Geometry: final body of the model. Coordinates: model frame, mm. A direction names the side the tool comes from. Coordinates: 2 decimals unless noted, no trailing zeros. Loops run counter-clockwise (first coordinate to the right, second up) from the corner with the lowest first, then second, coordinate; pieces in that order, holes last. Notation, with made-up numbers: (64, 52) -> (89, 52) arc R9 cw to (89, 64) -> close; hole circle Ø9 at (-16, 85). An arc over 180 degrees is marked (long way). One line per item, written item: value. Start each with the question number.
Item 1: Ray query, probe 1 along Y at (x, z) = (-123.5, -20.5) (1 decimal); probe 2 along Z at (x, y) = (-161, 75.5) (3 decimals); probe 3 along Y at (x, z) = (-197, 39) (1 decimal). Return the intervals inside material, ascending. Write a range as from..to.
Item 2: Set-up query: faces 5 (the flat face through (-121, 0, -2)), 6 (the flat face through (-190.5, 285, 1)), 7 (the flat face through (0, 237, -113)). Return all of +Z, -Z, +X, -X, +Y, -Y with unobstructed straight access to the full face (end or side cutting, diameter ignored); none if empty.
Item 3: Contact query for a flat-ended pin moving along its axis: pin 1 Ø3 at (y, z) = (298, 58) entering from +X. Output: stop coordinate, or through.
Item 4: Mould query, pull axis Y, two halves, no side actions, for faces 1 (the cylindrical face through (-143.266, 389.237, 132.457)), 2 (the flat face through (-137, 186, 139.7)), 3 (the flat face through (-122, 201, 104.775)), 4 (the flat face through (-247.65, 110, 1)). Classes: +Y half, -Y half, draft (parallel to the pull), parting line (faces both ways), or undercut.
Item 5: Section query B-B on y = 210. Return loops of the section in (x, z) (3 decimals), then the cut area to 3 significant figures.
Autodesk Inventor part; units mm, degrees
ref_plane "YZ Plane" through (0, 0, 0) normal (1, 0, 0) x (0, 1, 0)
ref_plane "XZ Plane" through (0, 0, 0) normal (0, 1, 0) x (-1, 0, 0)
ref_plane "XY Plane" through (0, 0, 0) normal (0, 0, 1) x (1, 0, 0)
sketch "Sketch1" plane through (0, 0, 0) normal (1, 0, 0) x (0, 1, 0)
  line L0 (0, 139.7) -> (396.875, 139.7)
  line L1 (396.875, 139.7) -> (396.875, -139.7)
  line L2 (396.875, -139.7) -> (0, -139.7)
  line L3 (0, -139.7) -> (0, 139.7)
  line L4 (396.875, -139.7) -> (0, 139.7) construction
  line L5 (23.8125, -104.775) -> (373.0625, -104.775)
  line L6 (373.0625, -104.775) -> (373.0625, 104.775)
  line L7 (373.0625, 104.775) -> (23.8125, 104.775)
  line L8 (23.8125, 104.775) -> (23.8125, -104.775)
  line L9 (23.8125, -104.775) -> (373.0625, 104.775) construction
  line L10 (373.0625, -104.775) -> (23.8125, 104.775) construction
  line L11 (23.8125, 104.775) -> (23.8125, 139.7)
  line L12 (23.8125, -104.775) -> (23.8125, -139.7)
  line L13 (198.4375, 104.775) -> (198.4375, -104.775)
  point P0 (0, 0)
  point P1 (0, 0)
  point P2 (198.4375, 0)
  dimension "d0" = 396.875
  dimension "d1" = 279.4
  dimension "d2" = 349.25
  dimension "d3" = 209.55
extrude "Extrusion1" add sketch "Sketch1" against normal blind 282.575
extrude "Extrusion2" add sketch "Sketch1" along normal blind 50.8 contours L0 L11 L8 L12 L2 L3
extrude "Extrusion3" cut sketch "Sketch1" against normal blind 190.5 contours L7 L6 L5 L13
extrude "Extrusion4" cut sketch "Sketch1" against normal blind 247.65 contours L7 L13 L5 L8
fillet "Fillet3" radius 38.1 2 edges at (50.8, 11.9063, -139.7) (50.8, 11.9062, 139.7)
fillet "Fillet1" radius 25.4 2 edges at (-141.2875, 396.875, 139.7) (-141.2875, 396.875, -139.7)
fillet "Fillet2" radius 6.35 2 edges at (-134.9375, 0, 139.7) (-134.9375, 0, -139.7)
properties part number "Fridge-Body"
Reply:
1. probe 1: y = 0..23.8, 373.1..396.9
1. probe 2: z = -139.7..-104.775, 104.775..139.7
1. probe 3: y = 0..23.8, 198.4..396.9
2. face 5: +Z, -Z, +X, -X, -Y
2. face 6: +X
2. face 7: +Z, -Z, +X, +Y
3. pin 1: stops at x = -190.5
4. face 1: +Y half
4. face 2: draft
4. face 3: undercut
4. face 4: undercut
5. outline: (-282.575, -139.7) -> (0, -139.7) -> (0, -104.775) -> (-190.5, -104.775) -> (-190.5, 104.775) -> (0, 104.775) -> (0, 139.7) -> (-282.575, 139.7) -> close
5. area: 39,000 mm²
